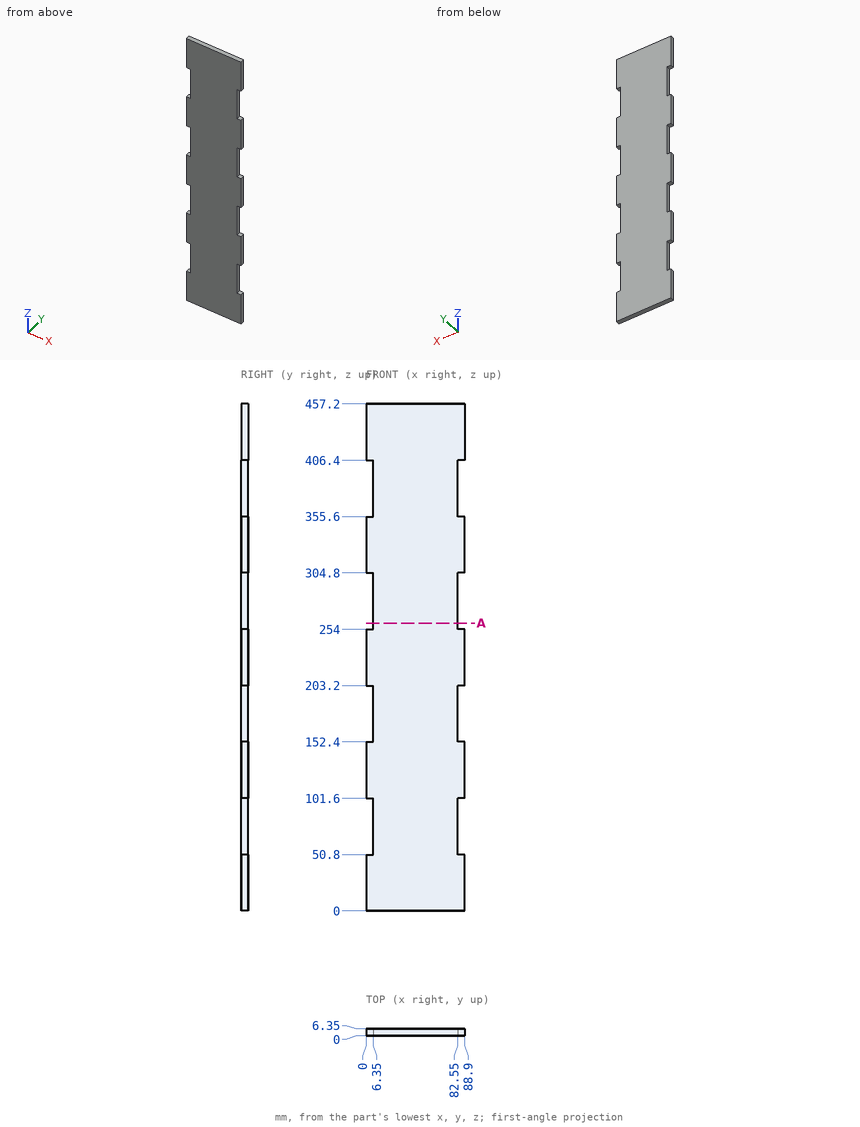
Geometry: see drawing. Coordinates: mm, zero at the bounding-box minimum. Coordinates: 2 decimals unless noted, no trailing zeros. Loops run counter-clockwise (first coordinate to the right, second up) from the corner with the lowest first, then second, coordinate; pieces in that order, holes last.
(1) Material intervals for probe 1 along Z at (x, y) = (85, 0.5); probe 2 along X at (y, z) = (1.25, 358), sorted ascending.
(2) First-contact query: pin 1 Ø3 at (y, z) = (2, 70.5) entering from +X; pin 2 Ø1.9 at (y, z) = (4.5, 87.5) entering from -X. Flat tips, straight axial feed; report the tip coordinate or a pass-through.
(3) Section A-A on z = 259.5. Return the cut outline in (x, y).
Data:
1. probe 1: z = 0 to 50.8, 101.6 to 152.4, 203.2 to 254, 304.8 to 355.6, 406.4 to 457.2
1. probe 2: x = 6.35 to 82.55
2. pin 1: stops at x = 82.55
2. pin 2: stops at x = 6.35
3. outline: (6.35, 0) - (82.55, 0) - (82.55, 6.35) - (6.35, 6.35) - close
